Check sheet for the modelled part. Datum: model origin and axes. Units: mm. A direction names the side the tool comes from. Give positions to 0.01 mm unless a question says otherwise; leave off trailing zeros. Write each loop counter-clockwise with the first axis right and the second up, starting at its lowest first coordinate (ties: lowest second). Pieces come first, ordered by that corner, then holes. Notation, with made-up numbers: M 34,36 L 84,36 A36 cw 84,75 Z; hole C 25,-11 d1. An arc over 180 degrees is marked long. Use CSV: the item, a comma, the result in double quotes. Start each with the question number.
1. Cross-section at B-B, the plane x = 0. Enter the section's corners in (y, z), and give its area (3 significant figures).
2. Cross-section at C-C, the plane z = -6.5. Enter the section's corners in (x, y).
3. Access from +Z, -Z, +X, -X, +Y, -Y to the whole of each face (thin tool, end or side, straight path). Record for faces 1 (the face through (-0.54, 4.93, 9.94)), 2 (the face through (-1.63, 5.14, -19.82)), 3 (the face through (-1.63, 6.04, 14.82)), 4 (the face through (3, 10, 7)).
4. Scan lines: line 1 (Z direction, x = 0, y = 5.25); line 2 (Z direction, x = 0, y = 3); line 3 (X direction, y = 2, z = 7.5). Record each from-to range of solid material in increasing order.
5. Depth check by flat-ended pin: P1, Ø1.5, axis at x = 4, z = -3, coming from the -Y side; P2, Ø5, axis at y = 5.5, z = -16.5, coming from the -X side; P3, Ø6.5, axis at x = 0, z = -12.5, coming from the -Y side; P4, Ø4, axis at x = -3, z = 0.5, coming from the +Y side. Enter the tip coordinate at first touch or a pass-through.
6. Mould release check, pull along X, two halves, no side actions. Record for faces 5 (the face through (-0.54, 5.14, -14.94)), 6 (the face through (7.5, 2, -3)), 7 (the face through (3, -5, -12)): +X half, -X half, draft (parallel to the pull), parting line (faces both ways), or undercut.
7. Cross-section at A-A, the plane y = 6. Enter the section's corners in (x, z), and give its area (3 significant figures).
8. Cross-section at D-D, the plane z = 1.5. Enter the section's corners in (x, y), and give its area (3 significant figures).
from build123d import *

# Parameters (mm, degrees)
CROQUIS3_R              = 2.5
SALIENTE_EXTRUIR1_DEPTH = 5
CROQUIS4_R              = 7.5
CROQUIS4_R_2            = 2.5
SALIENTE_EXTRUIR2_DEPTH = 5
CROQUIS5_R              = 7.5
CROQUIS5_R_2            = 2.5
SALIENTE_EXTRUIR3_DEPTH = 10
CROQUIS7_R              = 7.5
CROQUIS7_R_2            = 2.5
SALIENTE_EXTRUIR4_DEPTH = 5


with BuildPart() as part:
    # Croquis3 → Saliente-Extruir1 (new body)
    with BuildSketch(Plane(origin=(0, 0, 0), x_dir=(1, 0, 0), z_dir=(0, 1, 0))):
        with BuildLine():
            Line((-7.5, -7.5), (-7.5, 12.5))
            ThreePointArc((-7.5, 12.5), (0, 20), (7.5, 12.5))
            Line((7.5, 12.5), (7.5, -7.5))
            ThreePointArc((7.5, -7.5), (0, -15), (-7.5, -7.5))
        make_face()
        with Locations((0, 12.5)):
            Circle(CROQUIS3_R, mode=Mode.SUBTRACT)
        with Locations((0, -7.5)):
            Circle(CROQUIS3_R, mode=Mode.SUBTRACT)
    extrude(amount=SALIENTE_EXTRUIR1_DEPTH)

    # Croquis4 → Saliente-Extruir2 (add)
    with BuildSketch(Plane(origin=(0, 5, 0), x_dir=(1, 0, 0), z_dir=(0, 1, 0))):
        with Locations((0, -7.5)):
            Circle(CROQUIS4_R)
        with Locations((0, -7.5)):
            Circle(CROQUIS4_R_2, mode=Mode.SUBTRACT)
    extrude(amount=SALIENTE_EXTRUIR2_DEPTH)

    # Croquis5 → Saliente-Extruir3 (add)
    with BuildSketch(Plane(origin=(0, 5, 0), x_dir=(1, 0, 0), z_dir=(0, 1, 0))):
        with Locations((0, 12.5)):
            Circle(CROQUIS5_R)
        with Locations((0, 12.5)):
            Circle(CROQUIS5_R_2, mode=Mode.SUBTRACT)
    extrude(amount=SALIENTE_EXTRUIR3_DEPTH)

    # Croquis7 → Saliente-Extruir4 (add)
    with BuildSketch(Plane.XZ):
        with Locations((0, -12.5)):
            Circle(CROQUIS7_R)
        with Locations((0, -12.5)):
            Circle(CROQUIS7_R_2, mode=Mode.SUBTRACT)
    extrude(amount=SALIENTE_EXTRUIR4_DEPTH)


solid = part.part
Worked answers:
1,outline,"M -5,-20 L 15,-20 L 15,-15 L -5,-15 Z; M -5,-10 L 15,-10 L 15,-5 L 5,-5 L 5,0 L 10,0 L 10,5 L 0,5 L 0,-5 L -5,-5 Z; M 0,10 L 10,10 L 10,15 L 0,15 Z"
1,area,"325 mm^2"
2,outline,"M -7.5,0 L -4.5,0 L -4.5,-5 L 4.5,-5 L 4.5,0 L 7.5,0 L 7.5,5 L 4.5,5 L 4.5,15 L -4.5,15 L -4.5,5 L -7.5,5 Z"
3,face 1,"+Y, -Y"
3,face 2,"none"
3,face 3,"+Y"
3,face 4,"+Z, +X, -X, +Y"
4,line 1,"z = -20 to -15, -10 to -5, 0 to 5, 10 to 15"
4,line 2,"z = -20 to -15, -10 to 5, 10 to 15"
4,line 3,"x = -7.5 to -2.5, 2.5 to 7.5"
5,P1,"stops at y = 0"
5,P2,"stops at x = -7.35"
5,P3,"stops at y = -5"
5,P4,"stops at y = 10"
6,face 5,"undercut"
6,face 6,"+X half"
6,face 7,"draft"
7,outline,"C 0,-12.5 d15; C 0,7.5 d15; hole C 0,-12.5 d5; hole C 0,7.5 d5"
7,area,"314 mm^2"
8,outline,"M -7.5,0 L 7.5,0 L 7.5,5 L 4.5,5 L 4.5,10 L -4.5,10 L -4.5,5 L -7.5,5 Z"
8,area,"120 mm^2"
